Read the model definition and answer for the solid it produces. Units are mm, in the model's axes. Round coordinates to 2 decimals unless told otherwise and drop trailing zeros. Order: outer loops, then holes, each group sorted by start corner. A loop starts at its lowest first (then second) coordinate and runs counter-clockwise, first axis right, second up. Notation, with made-up numbers: (65, -28) - (85, -28) arc R19 ccw to (85, -4) - close; hole circle Ø2 at (-19.5, -17.5). An arc over 180 degrees is marked (long way). One line per question, with ' | ' between items. Start each with the question number.
1) The part is cut by section C-C, the plane y = 102.5. Give the vertices of the cut face in (x, z), plus the area to 3 significant figures.
2) The part is cut by section B-B, the plane y = 76.2. Give the vertices of the cut face in (x, z), plus the area to 3 significant figures.
3) Straight lines are drawn through the part: line 1 (Y direction, x = -30.5, z = 8.5); line 2 (X direction, y = 115, z = 5.25); line 3 (X direction, y = 153.5, z = 8). For each, find the intervals that lie inside material, in ascending order. Write a range as from..to.
4) The part is cut by section A-A, the plane z = 5.75. Give the vertices of the cut face in (x, y).
5) Flat-ended cylindrical pins translate along their axes: pin 1 (6.5 mm diameter, centred on y = 124, z = 5, fed in from -X); pin 2 (3 mm diameter, centred on y = 142.5, z = 4, fed in from +X); pin 3 (6.5 mm diameter, centred on y = 193, z = 6.5, fed in from +X). Find the tip coordinate at first contact, or state that the pin passes through.
6) The mould has two halves that part along X. Classify faces 1 (the cylindrical face through (-0.007, 76.864, 6.261)), 2 (the cylindrical face through (279.407, 75.533, 6.261)), 3 (the cylindrical face through (337.685, -3.033, 6.261)): pulls with the +X half, pulls with the -X half, needs draft (parallel to the pull), parting line crosses it, or undercut.
from build123d import *

# Parameters (mm, degrees)
F1_DEPTH = 12.7


with BuildPart() as f1:
    # F0 (on Top) → F1 (new body)
    with BuildSketch(Plane.XY):
        with BuildLine():
            ThreePointArc((-30.1752, 106.3752), (0, 76.2), (-30.1752, 46.0248))
            Line((-30.1752, 46.0248), (-30.1752, 16.449544))
            ThreePointArc((-30.1752, 16.449544), (-58.1152, -2.3876), (-30.1752, -21.224744))
            Line((-30.1752, -21.224744), (-30.1752, -50.8))
            Line((-30.1752, -50.8), (309.753, -50.8))
            Line((309.753, -50.8), (309.753, -21.313644))
            ThreePointArc((309.753, -21.313644), (337.693, -2.4765), (309.753, 16.360644))
            Line((309.753, 16.360644), (309.753, 45.847))
            ThreePointArc((309.753, 45.847), (279.4, 76.2), (309.753, 106.553))
            Line((309.753, 106.553), (309.753, 136.039356))
            ThreePointArc((309.753, 136.039356), (337.693, 154.8765), (309.753, 173.713644))
            Line((309.753, 173.713644), (309.753, 203.2))
            Line((309.753, 203.2), (-30.1752, 203.2))
            Line((-30.1752, 203.2), (-30.1752, 173.624744))
            ThreePointArc((-30.1752, 173.624744), (-58.1152, 154.7876), (-30.1752, 135.950456))
            Line((-30.1752, 135.950456), (-30.1752, 106.3752))
        make_face()
    extrude(amount=F1_DEPTH)


solid = f1.part
Values:
1) outline: (-15.38, 0) - (294.6, 0) - (294.6, 12.7) - (-15.38, 12.7) - close | area: 3,940 mm^2
2) outline: (0, 0) - (279.4, 0) - (279.4, 12.7) - (0, 12.7) - close | area: 3,550 mm^2
3) line 1: y = -21.35..16.58, 135.82..173.75 | line 2: x = -30.18..309.75 | line 3: x = -58.07..337.65
4) outline: (-30.18, -50.8) - (309.75, -50.8) - (309.75, -21.31) arc R20.32 ccw (long way) to (309.75, 16.36) - (309.75, 45.85) arc R30.35 cw to (309.75, 106.55) - (309.75, 136.04) arc R20.32 ccw (long way) to (309.75, 173.71) - (309.75, 203.2) - (-30.18, 203.2) - (-30.18, 173.62) arc R20.32 ccw (long way) to (-30.18, 135.95) - (-30.18, 106.38) arc R30.18 cw to (-30.18, 46.02) - (-30.18, 16.45) arc R20.32 ccw (long way) to (-30.18, -21.22) - close
5) pin 1: stops at x = -30.18 | pin 2: stops at x = 334.54 | pin 3: stops at x = 309.75
6) face 1: pulls with the -X half | face 2: pulls with the +X half | face 3: undercut
